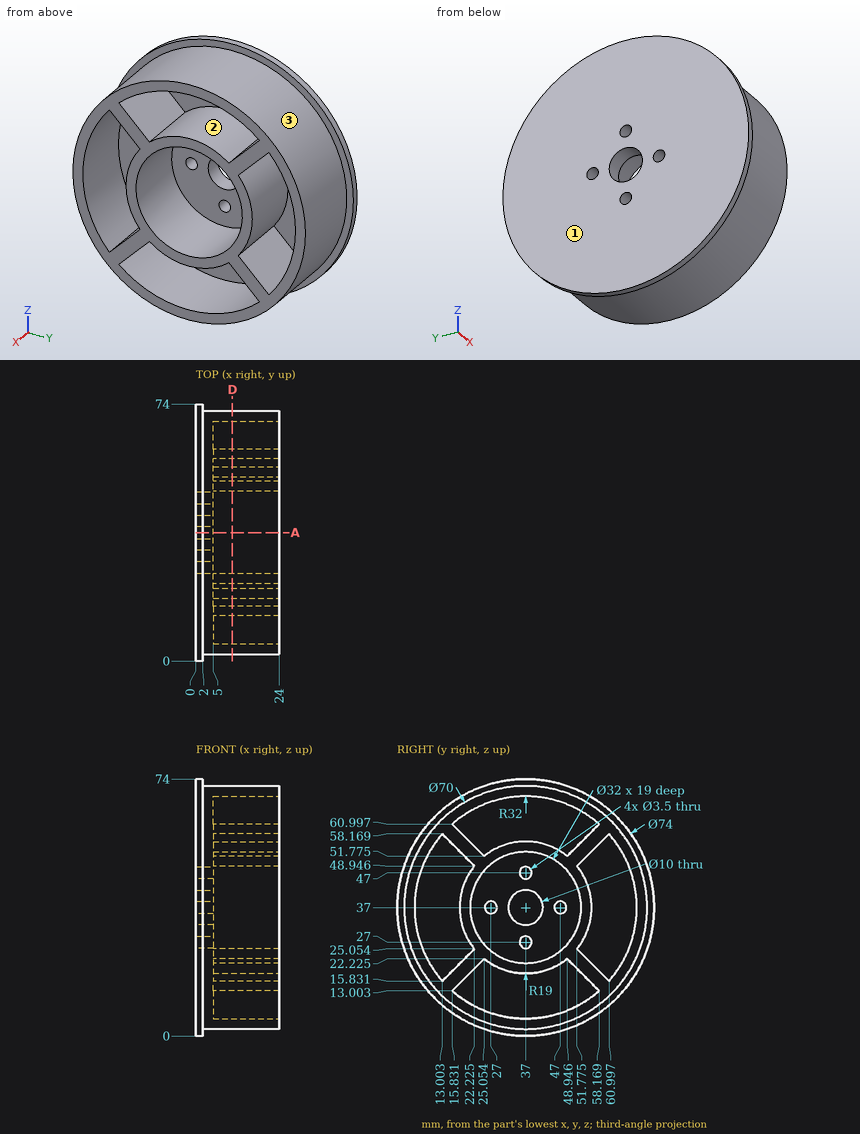
Verification items for this drawing (mm, ordinates from the low corner). Round coordinates to 2 decimals unless told otherwise and drop trailing zeros. Order: outer loops, then holes, each group sorted by start corner. A loop starts at its lowest first (then second) coordinate and runs counter-clockwise, first axis right, second up. Notation, with made-up numbers: (-19.5, -8.5) - (7.5, -8.5) arc R27 cw to (7.5, 14.5) - close; hole circle Ø9 at (51, 57.5). An arc over 180 degrees is marked (long way). Answer as CSV lines item,"result". Start each with the question number.
1) Draft check along Y on the marked faces 1, 2 and 3. Enter one of: +Y half, -Y half, draft (parallel to the pull), parting line (faces both ways), or undercut.
2) Depth check by flat-ended pin: pin 1 (1.5 mm diameter, centred on x = 19.5, z = 26.5, fed in from -Y) (1 decimal); pin 2 (4 mm diameter, centred on x = 7.5, z = 41, fed in from -Y); pin 3 (8 mm diameter, centred on x = 19, y = 49.5, fed in from +Z). Enter the tip coordinate at first touch or a pass-through.
3) Scan lines: probe 1 along Y at (x, z) = (1.45, 37); probe 2 along Y at (x, z) = (3.1, 37); probe 3 along Z at (x, y) = (18.5, 43.5) (1 decimal). Record each from-to range of solid material in increasing order.
4) Section check A-A (y = 37). Give the number of separate pieces and of enclosed holes in the cut face, then the cut area to 3 significant figures.
5) Section check D-D (x = 10.5). Record the cut outline in (y, z) (1 decimal), then the cut area to 3 significant figures.
Determined:
1,face 1,"draft"
1,face 2,"undercut"
1,face 3,"parting line"
2,pin 1,"y = 3.4"
2,pin 2,"y = 2.06"
2,pin 3,"z = 70.95"
3,probe 1,"0 to 25.25, 28.75 to 32, 42 to 45.25, 48.75 to 74"
3,probe 2,"2 to 25.25, 28.75 to 32, 42 to 45.25, 48.75 to 72"
3,probe 3,"2.6 to 5.7, 19.1 to 22.4, 51.6 to 54.9, 68.3 to 71.4"
4,separate pieces,"4"
4,enclosed holes,"0"
4,area,"501 mm^2"
5,outline,"circle Ø70 at (37, 37); hole (13, 15.8) - (22.2, 25.1) arc R19 cw to (22.2, 48.9) - (13, 58.2) arc R32 ccw to start; hole (15.8, 13) arc R32 ccw to (58.2, 13) - (48.9, 22.2) arc R19 cw to (25.1, 22.2) - close; hole (15.8, 61) - (25.1, 51.8) arc R19 cw to (48.9, 51.8) - (58.2, 61) arc R32 ccw to start; hole circle Ø32 at (37, 37); hole (51.8, 25.1) - (61, 15.8) arc R32 ccw to (61, 58.2) - (51.8, 48.9) arc R19 cw to start"
5,area,"1,170 mm^2"
